from build123d import *

# Parameters (mm, degrees)
SKETCH1_R           = 1.5
BOSS_EXTRUDE1_DEPTH = 6
SKETCH2_R           = 4.5
CUT_EXTRUDE1_DEPTH  = 2
SKETCH3_R           = 4
BOSS_EXTRUDE2_DEPTH = 7


with BuildPart() as part:
    # Sketch1 → Boss-Extrude1 (new body)
    with BuildSketch(Plane(origin=(0, 0, 0), x_dir=(1, 0, 0), z_dir=(0, 1, 0))):
        with BuildLine():
            Line((0, 6.5), (81, 6.5))
            ThreePointArc((81, 6.5), (84.25, 5.629165125), (86.629165125, 3.25))
            Line((86.629165125, 3.25), (102.629165125, -24.462812921))
            ThreePointArc((102.629165125, -24.462812921), (100.25, -33.341978046), (91.370834875, -30.962812921))
            Line((91.370834875, -30.962812921), (80.133974596, -11.5))
            ThreePointArc((80.133974596, -11.5), (76.473720558, -7.839745962), (71.473720558, -6.5))
            Line((71.473720558, -6.5), (0, -6.5))
            ThreePointArc((0, -6.5), (-6.5, 0), (0, 6.5))
        make_face()
        with Locations(Location((0, 0, 0), (0, 0, 270))):
            Circle(SKETCH1_R, mode=Mode.SUBTRACT)
        with Locations(Location((81, 0, 0), (0, 0, 270))):
            Circle(SKETCH1_R, mode=Mode.SUBTRACT)
    extrude(amount=BOSS_EXTRUDE1_DEPTH)

    # Sketch2 → Cut-Extrude1 (cut)
    with BuildSketch(Plane(origin=(0, 6, 0), x_dir=(1, 0, 0), z_dir=(0, 1, 0))):
        with Locations(Location((0, 0, 0), (0, 0, 270))):
            Circle(SKETCH2_R)
        with Locations(Location((81, 0, 0), (0, 0, 270))):
            Circle(SKETCH2_R)
    extrude(amount=-CUT_EXTRUDE1_DEPTH, mode=Mode.SUBTRACT)

    # Sketch3 → Boss-Extrude2 (add)
    with BuildSketch(Plane(origin=(0, 6, 0), x_dir=(1, 0, 0), z_dir=(0, 1, 0))):
        with Locations(Location((97, -27.712812921, 0), (0, 0, 270))):
            Circle(SKETCH3_R)
    extrude(amount=BOSS_EXTRUDE2_DEPTH)


solid = part.part
Part model, mm, in its own coordinate system. A direction names the side the tool comes from. Coordinates: 2 decimals unless noted, no trailing zeros. Loops run counter-clockwise (first coordinate to the right, second up) from the corner with the lowest first, then second, coordinate; pieces in that order, holes last. Notation, with made-up numbers: M 53.5,-11.5 L 103.5,-11.5 A10 cw 103.5,-4.5 Z; hole C 52.5,37.5 d6. An arc over 180 degrees is marked long. Use a Markdown table: item, result. Add a question column.
Q1. Cut at D-D (x = 65.5). Write the cut outline in (y, z).
Q2. Mould opens along X. For faces 1 (the flat face through (53, 0, 3)), 2 (the cylindrical face through (1.352, 5.014, 4.292)), 3 (the flat face through (85.831, 2.958, 21.368)), 4 (the cylindrical face through (85.46, 5.01, -0.59)) say: +X half, -X half, draft (parallel to the pull), parting line (faces both ways), or undercut.
Q3. Which spindle directions (+Z, -Z, +X, -X, +Y, -Y) get a long thin tool onto all of the face, cutting with end or side? Do faces 5 (the flat face through (36, 3, 6.5)), 6 (the cylindrical face through (93.095, 9.451, 26.846)), 7 (the cylindrical face through (100.37, 2.96, 33.27)). Say none if no direction does.
Q4. Pin check, flat tips, straight feed: P1, Ø2.5, axis at x = -1, z = 2, coming from the +Y side; P2, Ø5, axis at y = 5.5, z = 7, coming from the +X side; P3, Ø1.8, axis at x = 51, y = 3, coming from the +Z side. Stop position of each tip, or through.
Q5. Cut at B-B (z = 0). Write the cut outline in (x, y), and give its area (3 significant figures).
Q6. Cut at A-A (y = 2). Write the cut outline in (x, z).
Q7. Cut at C-C (y = 10). Write the cut outline in (x, z).
Q8. Probe L1, parallel to X at y = 4.85, z = 0; L2, parallel to Z at x = 81, y = 2.2; L3, parallel to X at y = 3, z = 0. List the from-to ranges inside material, lowest first.
Worked out:
| question | item | result |
|---|---|---|
| 1 | outline | M 0,-6.5 L 6,-6.5 L 6,6.5 L 0,6.5 Z |
| 2 | face 1 | draft |
| 2 | face 2 | undercut |
| 2 | face 3 | -X half |
| 2 | face 4 | undercut |
| 3 | face 5 | +Z, -X, +Y, -Y |
| 3 | face 6 | +Y |
| 3 | face 7 | +Y, -Y |
| 4 | P1 | stops at y = 4 |
| 4 | P2 | stops at x = 93.99 |
| 4 | P3 | stops at z = 6.5 |
| 5 | outline | M -6.5,0 L -1.5,0 L -1.5,4 L -4.5,4 L -4.5,6 L -6.5,6 Z; M 1.5,0 L 79.5,0 L 79.5,4 L 76.5,4 L 76.5,6 L 4.5,6 L 4.5,4 L 1.5,4 Z; M 82.5,0 L 88.51,0 L 88.51,6 L 85.5,6 L 85.5,4 L 82.5,4 Z |
| 5 | area | 510 mm2 |
| 6 | outline | M 0,-6.5 L 81,-6.5 A6.5 ccw 86.63,-3.25 L 102.63,24.46 A6.5 ccw 91.37,30.96 L 80.13,11.5 A10 cw 71.47,6.5 L 0,6.5 A6.5 ccw Z; hole C 0,0 d3; hole C 81,0 d3 |
| 7 | outline | C 97,27.71 d8 |
| 8 | L1 | x = -6.5 to -4.5, 4.5 to 76.5, 85.5 to 88.51 |
| 8 | L2 | z = -6.5 to -1.5, 1.5 to 13 |
| 8 | L3 | x = -6.5 to -1.5, 1.5 to 79.5, 82.5 to 88.51 |
